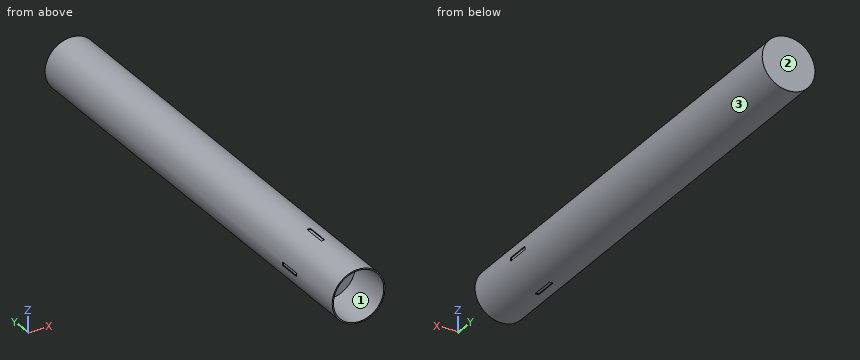
from build123d import *

# Parameters (mm, degrees)
SKETCH1_W           = 112
SKETCH1_H           = 2020
SKETCH2_W           = 15
SKETCH2_H           = 100
CUT_EXTRUDE1_DEPTH  = 132
SKETCH3_W           = 15
SKETCH3_H           = 100
BOSS_EXTRUDE1_DEPTH = 108
CIRPATTERN1_COUNT   = 4
SKETCH4_R           = 107
CUT_EXTRUDE2_DEPTH  = 200


with BuildPart() as part:
    # Sketch1 → Revolve1 (revolve)
    with BuildSketch(Plane.XY, mode=Mode.PRIVATE) as revolve1_sk:
        with Locations((56, -1010)):
            Rectangle(SKETCH1_W, SKETCH1_H)
    revolve(revolve1_sk.sketch.rotate(Axis((0, -2406.253229974, 0), (0, 1, 0)), 90), axis=Axis((0, -2406.253229974, 0), (0, 1, 0)))

    # Sketch2 → Cut-Extrude1 (cut)
    with BuildSketch(Plane.XY):
        with Locations((0, -1720)):
            Rectangle(SKETCH2_W, SKETCH2_H)
    cut_extrude1 = extrude(amount=-CUT_EXTRUDE1_DEPTH, mode=Mode.SUBTRACT)

    # Sketch3 → Boss-Extrude1 (add)
    with BuildSketch(Plane(origin=(0, 0, 0), x_dir=(-1, 0, 0), z_dir=(0, 0, -1))):
        with Locations((0, -1720)):
            Rectangle(SKETCH3_W, SKETCH3_H)
    boss_extrude1 = extrude(amount=BOSS_EXTRUDE1_DEPTH)

    # CirPattern1: Cut-Extrude1, Boss-Extrude1 ×4 about axis
    cirpattern1_axis = Axis((0, 0, 0), (0, 1, 0))
    add([cut_extrude1.rotate(cirpattern1_axis, i * 360 / CIRPATTERN1_COUNT) for i in range(1, CIRPATTERN1_COUNT)], mode=Mode.SUBTRACT)
    add([boss_extrude1.rotate(cirpattern1_axis, i * 360 / CIRPATTERN1_COUNT) for i in range(1, CIRPATTERN1_COUNT)])

    # Sketch4 → Cut-Extrude2 (cut)
    with BuildSketch(Plane.XZ.offset(2020)):
        with Locations(Location((0, 0, 0), (0, 0, 270))):
            Circle(SKETCH4_R)
    extrude(amount=-CUT_EXTRUDE2_DEPTH, mode=Mode.SUBTRACT)


solid = part.part
Geometry: final body of the model. Coordinates: model frame, mm. Face numbers are marked on the shaded views. Coordinates: 2 decimals unless noted, no trailing zeros. Order: outer loops, then holes, each group sorted by start corner. A loop starts at its lowest first (then second) coordinate and runs counter-clockwise, first axis right, second up.
(1) Section query B-B (y = -1743). Return the cut outline in (x, z).
(2) Section query C-C (x = 50). Return the cut outline in (y, z).
(3) Section query A-A (z = 89.5). Return the cut outline in (x, y).
(4) Material intervals for probe 1 along X at (y, z) = (-1961.5, 0); probe 2 along Y at (x, z) = (20, -37); probe 3 along X at (y, z) = (-1850.5, 58), sorted ascending.
(5) Draft query along X for the marked faces 1, 2 and 3. Return one class per face: pulls with the +X half, pulls with the -X half, needs draft (parallel to the pull), parting line crosses it, or undercut.
(6) First-contact query: pin 1 (12 mm diameter, centred on x = -88.5, z = 50.5, fed in from +Y); pin 2 (3 mm diameter, centred on x = 47, y = -1377.5, fed in from +Z); pin 3 (7.5 mm diameter, centred on y = -1732, z = 0, fed in from +X); pin 4 (3 mm diameter, centred on x = 60.5, y = -1000, fed in from -Z). Flat tips, straight axial feed; report the tip coordinate or a pass-through.
Solution:
1. outline: (-111.75, -7.5) arc R112 ccw to (-7.5, -111.75) - (-7.5, -108) - (7.5, -108) - (7.5, -111.75) arc R112 ccw to (111.75, -7.5) - (108, -7.5) - (108, 7.5) - (111.75, 7.5) arc R112 ccw to (7.5, 111.75) - (7.5, 108) - (-7.5, 108) - (-7.5, 111.75) arc R112 ccw to (-111.75, 7.5) - (-108, 7.5) - (-108, -7.5) - close
2. outline: (-2020, -100.22) - (0, -100.22) - (0, 100.22) - (-2020, 100.22) - (-2020, 94.6) - (-1820, 94.6) - (-1820, -94.6) - (-2020, -94.6) - close
3. outline: (-67.33, -2020) - (-58.64, -2020) - (-58.64, -1820) - (58.64, -1820) - (58.64, -2020) - (67.33, -2020) - (67.33, 0) - (-67.33, 0) - close
4. probe 1: x = -112 to -107, 107 to 112
4. probe 2: y = -1820 to 0
4. probe 3: x = -95.81 to -89.92, 89.92 to 95.81
5. face 1: undercut
5. face 2: needs draft
5. face 3: parting line crosses it
6. pin 1: stops at y = 0
6. pin 2: stops at z = 102.34
6. pin 3: stops at x = 108
6. pin 4: stops at z = -95.2
